```python
from build123d import *

# Parameters (mm, degrees)
SKETCH_1_W          = 60
SKETCH_1_H          = 40
SKETCH_1_R          = 7.5
SKETCH_1_R_2        = 2
EXTRUDE_1_DEPTH     = 4
EXTRUDE_2_DEPTH     = 4
SKETCH_6_W          = 4
SKETCH_6_H          = 68.008301528
EXTRUDE_3_DEPTH     = 60
SKETCH_7_R          = 2.5
CUT_EXTRUDE_1_DEPTH = 114.512737176
FILLET_1_R          = 10
FILLET_2_R          = 20
FILLET_4_R          = 10
FILLET_12_R         = 0.5
FILLET_13_R         = 0.5
SKETCH_10_W         = 25
SKETCH_10_H         = 3
EXTRUDE_6_DEPTH     = 75
FILLET_16_R         = 10


with BuildPart() as part:
    # 草图1 → 凸台-拉伸1 (new body)
    with BuildSketch(Plane(origin=(0, 0, 0), x_dir=(1, 0, 0), z_dir=(0, 1, 0))):
        with Locations((-43.629618652, 19.709362445)):
            Rectangle(SKETCH_1_W, SKETCH_1_H)
        with Locations(Location((-33.629618652, 19.709362445, 0), (0, 0, 270))):
            Circle(SKETCH_1_R, mode=Mode.SUBTRACT)
        with Locations(Location((-42.822006808, 28.9017506, 0), (0, 0, 270))):
            Circle(SKETCH_1_R_2, mode=Mode.SUBTRACT)
        with Locations(Location((-24.437230497, 28.9017506, 0), (0, 0, 270))):
            Circle(SKETCH_1_R_2, mode=Mode.SUBTRACT)
        with Locations(Location((-24.437230497, 10.516974289, 0), (0, 0, 270))):
            Circle(SKETCH_1_R_2, mode=Mode.SUBTRACT)
        with Locations(Location((-42.822006808, 10.516974289, 0), (0, 0, 270))):
            Circle(SKETCH_1_R_2, mode=Mode.SUBTRACT)
    extrude(amount=EXTRUDE_1_DEPTH)

    # 草图2 → 凸台-拉伸2 (add)
    with BuildSketch(Plane.ZY.offset(73.629618652)):
        Polygon((-53.713513209, 20), (-39.709362445, 0), (0.290637555, 0), (14.294788319, 20), align=None)
    extrude(amount=EXTRUDE_2_DEPTH)

    # 草图6 → 凸台-拉伸3 (add)
    with BuildSketch(Plane(origin=(0, 20, 0), x_dir=(1, 0, 0), z_dir=(0, 1, 0))):
        with Locations((-75.629618652, 19.709362445)):
            Rectangle(SKETCH_6_W, SKETCH_6_H)
    extrude(amount=EXTRUDE_3_DEPTH)

    # 草图7 → 切除-拉伸1 (cut, through all)
    with BuildSketch(Plane(origin=(-73.629618652, 0, 0), x_dir=(0, 0, -1), z_dir=(1, 0, 0))):
        with Locations((48.713513209, 25)):
            Circle(SKETCH_7_R)
        with Locations((-9.286486791, 25)):
            Circle(SKETCH_7_R)
        with Locations((48.713513209, 70)):
            Circle(SKETCH_7_R)
        with Locations((-9.286486791, 70)):
            Circle(SKETCH_7_R)
    extrude(amount=-CUT_EXTRUDE_1_DEPTH, mode=Mode.SUBTRACT)

    # 圆角1
    fillet_1_edges = [part.edges().sort_by_distance(p)[0] for p in [
        (-13.629618652, 2, -39.709362445),
        (-13.629618652, 2, 0.290637555),
    ]]
    fillet(fillet_1_edges, radius=FILLET_1_R)

    # 圆角2
    fillet_2_edges = [part.edges().sort_by_distance(p)[0] for p in [
        (-75.629618652, 20, 14.294788319),
        (-75.629618652, 20, -53.713513209),
    ]]
    fillet(fillet_2_edges, radius=FILLET_2_R)

    # 圆角4
    fillet_4_edges = [part.edges().sort_by_distance(p)[0] for p in [
        (-75.629618652, 80, -53.713513209),
        (-75.629618652, 80, 14.294788319),
    ]]
    fillet(fillet_4_edges, radius=FILLET_4_R)

    # 圆角12
    fillet_12_edges = [part.edges().sort_by_distance(p)[0] for p in [
        (-73.629618652, 80, -19.709362445),
        (-73.629618652, 48.152987889, -53.713513209),
        (-73.629618652, 48.152987889, 14.294788319),
        (-73.629618652, 77.071067812, -50.784581021),
        (-73.629618652, 77.071067812, 11.365856131),
        (-73.629618652, 7.417223525, 5.48423338),
        (-73.629618652, 7.417223525, -44.90295827),
        (-73.629618652, 20.291859787, 13.369127334),
        (-73.629618652, 20.291859787, -52.787852224),
    ]]
    fillet(fillet_12_edges, radius=FILLET_12_R)

    # 圆角13
    fillet_13_edges = [part.edges().sort_by_distance(p)[0] for p in [
        (-77.629618652, 80, -19.709362445),
        (-77.629618652, 48.152987889, 14.294788319),
        (-77.629618652, 48.152987889, -53.713513209),
        (-77.629618652, 77.071067812, -50.784581021),
        (-77.629618652, 77.071067812, 11.365856131),
        (-77.629618652, 7.417223525, 5.48423338),
        (-77.629618652, 7.417223525, -44.90295827),
        (-77.629618652, 20.291859787, 13.369127334),
        (-77.629618652, 20.291859787, -52.787852224),
    ]]
    fillet(fillet_13_edges, radius=FILLET_13_R)

    # 草图10 → 凸台-拉伸6 (add)
    with BuildSketch(Plane(origin=(0, 4, 0), x_dir=(1, 0, 0), z_dir=(0, 1, 0))):
        with Locations((-61.129618652, 38.209362445)):
            Rectangle(SKETCH_10_W, SKETCH_10_H)
        with Locations((-61.129618652, 1.209362445)):
            Rectangle(SKETCH_10_W, SKETCH_10_H)
    extrude(amount=EXTRUDE_6_DEPTH)

    # 圆角16
    fillet_16_edges = [part.edges().sort_by_distance(p)[0] for p in [
        (-48.629618652, 79, -38.209362445),
        (-48.629618652, 79, -1.209362445),
    ]]
    fillet(fillet_16_edges, radius=FILLET_16_R)


solid = part.part
```
The model under review builds one solid part; all positions refer to its coordinate system, in mm. A direction names the side the tool comes from. Round coordinates to 2 decimals unless told otherwise and drop trailing zeros. Loops run counter-clockwise (first coordinate to the right, second up) from the corner with the lowest first, then second, coordinate; pieces in that order, holes last. Notation, with made-up numbers: M 9,38 L 52,38 A20 cw 52,70 Z; hole C -4.75,-1.75 d3. An arc over 180 degrees is marked long. Put each result on its own line as item: value.
Q1. Consider section D-D, the plane y = 25. Count the separate pieces of the cut face and the enclosed holes in it, then the cut area to 3 significant figures.
Result set:
separate pieces: 3
enclosed holes: 0
area: 381 mm²
Q2. Consider section B-B, the plane y = 40. Give the boundary of the cut face in (x, z).
Result set:
outline: M -77.63,-53.21 A0.5 ccw -77.13,-53.71 L -74.13,-53.71 A0.5 ccw -73.63,-53.21 L -73.63,-39.71 L -48.63,-39.71 L -48.63,-36.71 L -73.63,-36.71 L -73.63,-2.71 L -48.63,-2.71 L -48.63,0.29 L -73.63,0.29 L -73.63,13.79 A0.5 ccw -74.13,14.29 L -77.13,14.29 A0.5 ccw -77.63,13.79 Z
Q3. Consider section C-C, the plane z = -6.5. Give the boundary of the cut face in (x, y), then the cut area to 3 significant figures.
Result set:
outline: M -77.63,0 L -14.16,0 L -14.16,4 L -73.63,4 L -73.63,79.5 A0.5 ccw -74.13,80 L -77.13,80 A0.5 ccw -77.63,79.5 Z
area: 558 mm²
Q4. To check wall thickness, follow L1, parallel to Z at x = -55, y = 18; L2, parallel to Y at x = -74, z = -47.5; L3, parallel to X at y = 27, z = 6. State the ranges of each line that lie inside material, in increasing order.
Result set:
L1: z = -39.71 to -36.71, -2.71 to 0.29
L2: y = 11.16 to 22.81, 27.19 to 67.81, 72.19 to 79.24
L3: x = -77.63 to -73.63
Q5. Consider section A-A, the plane x = -69. Give the boundary of the cut face in (y, z), then the cut area to 3 significant figures.
Result set:
outline: M 0,-39.71 L 79,-39.71 L 79,-36.71 L 4,-36.71 L 4,-2.71 L 79,-2.71 L 79,0.29 L 0,0.29 Z
area: 610 mm²
Q6. Mouldability with a two-part tool opening along Y and no side actions: class faces 3 (the cylindrical face through (-75.6, 27.48, 9.61)), 4 (the flat face through (-66, 79, -1)), 5 (the flat face through (-61, 41, -2.709)) as released by +Y, released by -Y, zero draft, split by the parting line, or undercut.
Result set:
face 3: undercut
face 4: released by +Y
face 5: zero draft
Q7. Machinability: for faces 1 (the flat face through (-48.63, 36, -38)), 2 (the flat face through (-75.609, 7.521, -44.976)), which of the approach directions +Z, -Z, +X, -X, +Y, -Y give a long, thin tool a straight path to every point of the face, cutting with its end or side? Answer none if there is none.
Result set:
face 1: +Z, -Z, +X, +Y
face 2: -Z, +X, -X, -Y
Q8. For pin 1 (8 mm diameter, centred on x = -52, y = 8.5, fed in from -Z); pin 2 (1.5 mm diameter, centred on x = -63.5, z = -39, fed in from +Y); pin 3 (1 mm diameter, centred on x = -37.5, z = -23.5, fed in from -Y); pin 4 (5 mm diameter, centred on y = 43.5, z = -32.5, fed in from +X), all flat-tipped, find the tip position at first contact; note any pin that passes through.
Result set:
pin 1: stops at z = -39.71
pin 2: stops at y = 79
pin 3: passes through
pin 4: stops at x = -73.63
